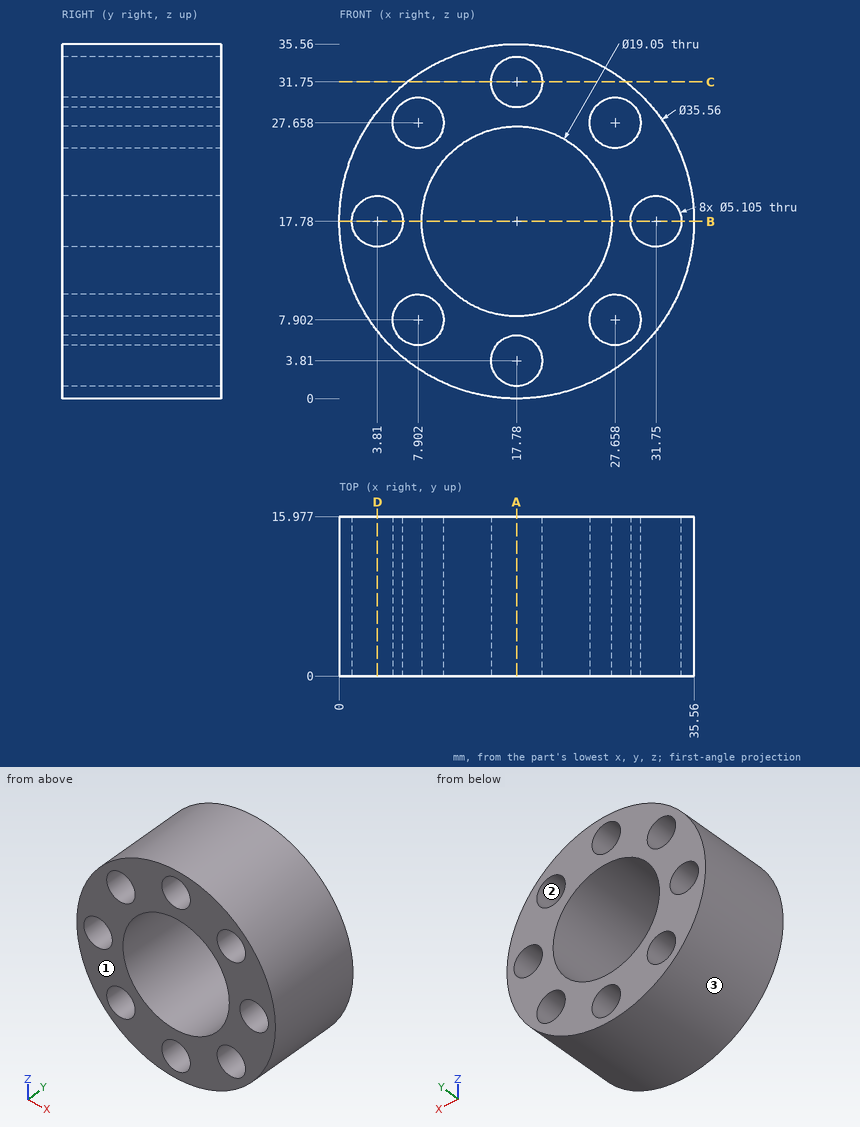
Could you check a few things on this drawing? It's one solid part, dimensions in mm from its lowest x, y, z. Round coordinates to 2 decimals unless told otherwise and drop trailing zeros. Loops run counter-clockwise (first coordinate to the right, second up) from the corner with the lowest first, then second, coordinate; pieces in that order, holes last. Notation, with made-up numbers: (-1, 25.5) -> (53, 25.5) arc R36 cw to (53, 63.5) -> close; hole circle Ø6 at (21, 4.25). An arc over 180 degrees is marked (long way). Write each question's results on one line, items separated by ' | '.
(1) If we section it at D-D, the plane x = 3.81: List the corners of the cut face in (y, z) for me, then the cut area to 3 significant figures.
Worked answers:
outline: (0, 6.78) -> (15.98, 6.78) -> (15.98, 15.23) -> (0, 15.23) -> close; (0, 20.33) -> (15.98, 20.33) -> (15.98, 28.78) -> (0, 28.78) -> close | area: 270 mm2
(2) If we section it at A-A, the plane x = 17.78: List the corners of the cut face in (y, z) for me (1 decimal), then the cut area to 3 significant figures.
Worked answers:
outline: (0, 0) -> (16, 0) -> (16, 1.3) -> (0, 1.3) -> close; (0, 6.4) -> (16, 6.4) -> (16, 8.3) -> (0, 8.3) -> close; (0, 27.3) -> (16, 27.3) -> (16, 29.2) -> (0, 29.2) -> close; (0, 34.3) -> (16, 34.3) -> (16, 35.6) -> (0, 35.6) -> close | area: 101 mm2
(3) For P1, Ø8, axis at x = 27.66, z = 7.9, coming from the +Y side; P2, Ø1.5, axis at y = 11.5, z = 7, coming from the +X side; P3, Ø4, axis at x = 17.78, z = 31.75, coming from the -Y side; P4, Ø3, axis at x = 14, y = 12, coming from the +Z side, each with a flat end and sliding along its axis, tell me the tip position at first contact or that it passes through.
Worked answers:
P1: y = 15.98 | P2: x = 32.46 | P3: through | P4: z = 35.41
(4) If I drill on L1, parallel to X at y = 8.5, z = 17.78 (1 decimal); L2, parallel to Z at x = 30, y = 5 (1 decimal); L3, parallel to Z at x = 7, y = 7.75 (1 decimal), over which ranges is the centre line in solid material (lowest first)?
Worked answers:
L1: 0 to 1.3, 6.4 to 8.3, 27.3 to 29.2, 34.3 to 35.6 | L2: 4.9 to 6.9, 8.9 to 15.9, 19.6 to 26.6, 28.7 to 30.7 | L3: 3.6 to 5.5, 10.3 to 25.3, 30 to 31.9
(5) We'd pull the mould along Z, two halves only. Please class the marked faces 1, 2 and 3: released by +Z, released by -Z, zero draft, split by the parting line, or undercut.
Worked answers:
face 1: zero draft | face 2: undercut | face 3: split by the parting line
(6) If we section it at C-C, the plane z = 31.75: List the corners of the cut face in (x, y) for me, then the cut area to 3 significant figures.
Worked answers:
outline: (6.78, 0) -> (15.23, 0) -> (15.23, 15.98) -> (6.78, 15.98) -> close; (20.33, 0) -> (28.78, 0) -> (28.78, 15.98) -> (20.33, 15.98) -> close | area: 270 mm2
(7) If we section it at B-B, the plane z = 17.78: List the corners of the cut face in (x, y) for me (1 decimal), then the cut area to 3 significant figures.
Worked answers:
outline: (0, 0) -> (1.3, 0) -> (1.3, 16) -> (0, 16) -> close; (6.4, 0) -> (8.3, 0) -> (8.3, 16) -> (6.4, 16) -> close; (27.3, 0) -> (29.2, 0) -> (29.2, 16) -> (27.3, 16) -> close; (34.3, 0) -> (35.6, 0) -> (35.6, 16) -> (34.3, 16) -> close | area: 101 mm2
